Source: CAD feature listing. Evaluate the final solid. Frame: model axes, mm. Face numbers are marked on the shaded views. A direction names the side the tool comes from. Coordinates: 2 decimals unless noted, no trailing zeros. Loops run counter-clockwise (first coordinate to the right, second up) from the corner with the lowest first, then second, coordinate; pieces in that order, holes last.
from build123d import *

# Parameters (mm, degrees)
CORTAR_EXTRUIR1_DEPTH = 89.610326763


with BuildPart() as part:
    # Croquis2 → Revolución1 (revolve)
    with BuildSketch(Plane.XY):
        with BuildLine():
            Line((3.175, 70), (12.7, 70))
            Line((12.7, 70), (12.7, 87.7))
            add(Edge.make_bspline(
                [(12.7, 87.7), (18.502741551, 87.7), (18.502741551, 82.7)],
                knots=[0, 0, 0, 1, 1, 1], degree=2))
            Line((18.502741551, 82.7), (22.5, 82.7))
            Line((22.5, 82.7), (22.5, 87.7))
            add(Edge.make_bspline(
                [(7.5, 102.7), (13.042740157, 102.7), (19.451979538, 97.810764177), (22.5, 90.380625461), (22.5, 87.7)],
                knots=[0, 0, 0, 0, 0.655380699, 1, 1, 1, 1], degree=3))
            Line((7.5, 102.7), (7.5, 90))
            Line((7.5, 90), (0, 90))
            Line((0, 90), (0, 0))
            Line((0, 0), (6.35, 0))
            Line((6.35, 0), (6.35, 3))
            Line((6.35, 3), (4.175, 4.255736835))
            Line((4.175, 4.255736835), (3.175, 4.255736835))
            Line((3.175, 4.255736835), (3.175, 70))
        make_face()
    revolve(axis=Axis((0, 0, 0), (0, 1, 0)))

    # Croquis3 → Cortar-Extruir1 (cut, through all)
    with BuildSketch(Plane.XZ.offset(-82.7)):
        with BuildLine():
            ThreePointArc((20.772727273, 8.645449766), (19.5, 0), (20.772727273, -8.645449766))
            ThreePointArc((20.772727273, -8.645449766), (22.5, 0), (20.772727273, 8.645449766))
        make_face()
        with BuildLine():
            ThreePointArc((17.873542761, -13.666984641), (9.75, -16.887495374), (2.899184512, -22.312434407))
            ThreePointArc((2.899184512, -22.312434407), (11.25, -19.485571585), (17.873542761, -13.666984641))
        make_face()
        with BuildLine():
            ThreePointArc((-2.899184512, -22.312434407), (-9.75, -16.887495374), (-17.873542761, -13.666984641))
            ThreePointArc((-17.873542761, -13.666984641), (-11.25, -19.485571585), (-2.899184512, -22.312434407))
        make_face()
        with BuildLine():
            ThreePointArc((-20.772727273, -8.645449766), (-19.5, 0), (-20.772727273, 8.645449766))
            ThreePointArc((-20.772727273, 8.645449766), (-22.5, 0), (-20.772727273, -8.645449766))
        make_face()
        with BuildLine():
            ThreePointArc((-17.873542761, 13.666984641), (-9.75, 16.887495374), (-2.899184512, 22.312434407))
            ThreePointArc((-2.899184512, 22.312434407), (-11.25, 19.485571585), (-17.873542761, 13.666984641))
        make_face()
        with BuildLine():
            ThreePointArc((2.899184512, 22.312434407), (9.75, 16.887495374), (17.873542761, 13.666984641))
            ThreePointArc((17.873542761, 13.666984641), (11.25, 19.485571585), (2.899184512, 22.312434407))
        make_face()
    extrude(amount=-CORTAR_EXTRUIR1_DEPTH, mode=Mode.SUBTRACT)


solid = part.part
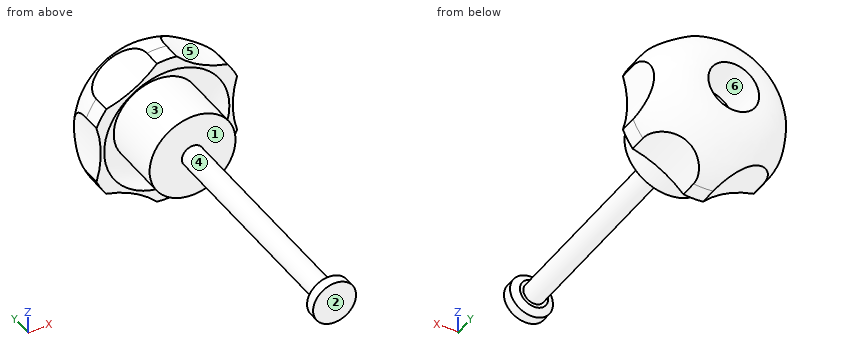
Q1. Line query: line 1 along X through (y, z) = (93, 0); line 2 along Z through (x, y) = (0, 97.25); line 3 along Y through (x, z) = (4, 0.5). Output: solid intervals per line, ascending.
Q2. Section B-B, the plane y = 77.5. Return the cut outline in (x, z).
Q3. Draft query along Y for the marked faces 1, 2 and 3. Return one class per face: +Y half, -Y half, draft (parallel to the pull), parting line (faces both ways), or undercut.
Q4. Section A-A, the plane y = 37. Return the cut outline in (x, z) (3 decimals).
Q5. Access query for the marked faces 4, 5 and 6. Directions: +Z, -Z, +X, -X, +Y, -Y. A direction counts if a zero-diameter tool reaches every point of the face in a straight line with its end or side. Return the directions, or none.
Q6. Contact query for flat-ended pins moving along their axis: pin 1 Ø12 at (x, y) = (3, 87) entering from -Z; pin 2 Ø6 at (x, y) = (-8.5, 23) entering from +Z; pin 3 Ø2.5 at (x, z) = (-0.5, -0.5) entering from +Y; pin 4 Ø3 at (x, y) = (2, 88) entering from +Z. Output: stop coordinate, or through.
Derived:
1. line 1: x = -19.5 to -7.5, 7.5 to 19.5
1. line 2: z = -18.5 to -7.5, 7.5 to 18.5
1. line 3: y = 0 to 4.26, 70 to 90
2. outline: circle Ø25.4 at (0, 0)
3. face 1: undercut
3. face 2: -Y half
3. face 3: draft
4. outline: circle Ø6.35 at (0, 0)
5. face 4: none
5. face 5: +Z, +X, +Y, -Y
5. face 6: +Y
6. pin 1: stops at z = -22.5
6. pin 2: passes through
6. pin 3: stops at y = 90
6. pin 4: stops at z = 22.49
